```python
from build123d import *

# Parameters (mm, degrees)
F0_R     = 44.45
F0_R_2   = 6.35
F1_DEPTH = 3.175


with BuildPart() as f1:
    # F0 (on Top) → F1 (new body)
    with BuildSketch(Plane.XY):
        Circle(F0_R)
        with BuildLine():
            add(Edge.make_bspline(
                [(-20.4392500678, -2.7074250448), (-18.5086635833, -4.8096192168), (-18.5086635833, -8.1559691232)],
                knots=[0, 0, 0, 1, 1, 1], degree=2))
            add(Edge.make_bspline(
                [(-18.5086635833, -8.1559691232), (-18.5086635833, -12.4676122719), (-21.6369287203, -14.8844205377)],
                knots=[0, 0, 0, 1, 1, 1], degree=2))
            add(Edge.make_bspline(
                [(-21.6369287203, -14.8844205377), (-24.7651938572, -17.3012288034), (-30.1279340918, -17.3012288034)],
                knots=[0, 0, 0, 1, 1, 1], degree=2))
            add(Edge.make_bspline(
                [(-30.1279340918, -17.3012288034), (-35.9339941859, -17.3012288034), (-39.065834483, -15.7996615377)],
                knots=[0, 0, 0, 1, 1, 1], degree=2))
            Line((-39.065834483, -15.7996615377), (-39.065834483, -12.1386975375))
            add(Edge.make_bspline(
                [(-39.065834483, -12.1386975375), (-37.0494441547, -12.9824353344), (-34.6826881312, -13.475807436)],
                knots=[0, 0, 0, 1, 1, 1], degree=2))
            add(Edge.make_bspline(
                [(-34.6826881312, -13.475807436), (-32.3159321076, -13.9691795376), (-29.9920780059, -13.9691795376)],
                knots=[0, 0, 0, 1, 1, 1], degree=2))
            add(Edge.make_bspline(
                [(-29.9920780059, -13.9691795376), (-26.1952579197, -13.9691795376), (-24.2718217556, -12.5283899946)],
                knots=[0, 0, 0, 1, 1, 1], degree=2))
            add(Edge.make_bspline(
                [(-24.2718217556, -12.5283899946), (-22.3483855914, -11.0876004515), (-22.3483855914, -8.5134851389)],
                knots=[0, 0, 0, 1, 1, 1], degree=2))
            add(Edge.make_bspline(
                [(-22.3483855914, -8.5134851389), (-22.3483855914, -6.8188592247), (-23.0312411813, -5.7355856973)],
                knots=[0, 0, 0, 1, 1, 1], degree=2))
            add(Edge.make_bspline(
                [(-23.0312411813, -5.7355856973), (-23.7140967712, -4.6523121699), (-25.3121933611, -3.7334960097)],
                knots=[0, 0, 0, 1, 1, 1], degree=2))
            add(Edge.make_bspline(
                [(-25.3121933611, -3.7334960097), (-26.910289951, -2.8146798495), (-30.1708360137, -1.6563279588)],
                knots=[0, 0, 0, 1, 1, 1], degree=2))
            add(Edge.make_bspline(
                [(-30.1708360137, -1.6563279588), (-34.725590053, -0.0260549274), (-36.6812026586, 2.2084201704)],
                knots=[0, 0, 0, 1, 1, 1], degree=2))
            add(Edge.make_bspline(
                [(-36.6812026586, 2.2084201704), (-38.6368152642, 4.4428952681), (-38.6368152642, 8.0395063855)],
                knots=[0, 0, 0, 1, 1, 1], degree=2))
            add(Edge.make_bspline(
                [(-38.6368152642, 8.0395063855), (-38.6368152642, 11.8148755108), (-35.8017132601, 14.0493506086)],
                knots=[0, 0, 0, 1, 1, 1], degree=2))
            add(Edge.make_bspline(
                [(-35.8017132601, 14.0493506086), (-32.9666112561, 16.2838257063), (-28.2903017714, 16.2838257063)],
                knots=[0, 0, 0, 1, 1, 1], degree=2))
            add(Edge.make_bspline(
                [(-28.2903017714, 16.2838257063), (-23.4209336383, 16.2838257063), (-19.3309504193, 14.4962456281)],
                knots=[0, 0, 0, 1, 1, 1], degree=2))
            Line((-19.3309504193, 14.4962456281), (-20.5179035913, 11.1927976435))
            add(Edge.make_bspline(
                [(-20.5179035913, 11.1927976435), (-24.5649848884, 12.8874235577), (-28.3832559355, 12.8874235577)],
                knots=[0, 0, 0, 1, 1, 1], degree=2))
            add(Edge.make_bspline(
                [(-28.3832559355, 12.8874235577), (-31.4006911075, 12.8874235577), (-33.0988921819, 11.5932155811)],
                knots=[0, 0, 0, 1, 1, 1], degree=2))
            add(Edge.make_bspline(
                [(-33.0988921819, 11.5932155811), (-34.7970932562, 10.2990076044), (-34.7970932562, 7.9966044637)],
                knots=[0, 0, 0, 1, 1, 1], degree=2))
            add(Edge.make_bspline(
                [(-34.7970932562, 7.9966044637), (-34.7970932562, 6.3019785495), (-34.1714402288, 5.2151298619)],
                knots=[0, 0, 0, 1, 1, 1], degree=2))
            add(Edge.make_bspline(
                [(-34.1714402288, 5.2151298619), (-33.5457872014, 4.1282811744), (-32.0585205763, 3.2237656548)],
                knots=[0, 0, 0, 1, 1, 1], degree=2))
            add(Edge.make_bspline(
                [(-32.0585205763, 3.2237656548), (-30.5712539512, 2.3192501352), (-27.5109168573, 1.2252511273)],
                knots=[0, 0, 0, 1, 1, 1], degree=2))
            add(Edge.make_bspline(
                [(-27.5109168573, 1.2252511273), (-22.3698365523, -0.6052308728), (-20.4392500678, -2.7074250448)],
                knots=[0, 0, 0, 1, 1, 1], degree=2))
        make_face(mode=Mode.SUBTRACT)
        Polygon((-1.7697637308, 12.4441036983), (-1.7697637308, -16.8507586237), (-5.566583817, -16.8507586237), (-5.566583817, 12.4441036983), (-15.9130973098, 12.4441036983), (-15.9130973098, 15.819054886), (8.576749762, 15.819054886), (8.576749762, 12.4441036983), align=None, mode=Mode.SUBTRACT)
        with BuildLine():
            Line((34.3679551307, 15.819054886), (38.1647752168, 15.819054886))
            Line((38.1647752168, 15.819054886), (38.1647752168, -5.317291959))
            add(Edge.make_bspline(
                [(38.1647752168, -5.317291959), (38.1647752168, -10.9088424437), (34.7898240291, -14.1050356236)],
                knots=[0, 0, 0, 1, 1, 1], degree=2))
            add(Edge.make_bspline(
                [(34.7898240291, -14.1050356236), (31.4148728414, -17.3012288034), (25.5158585833, -17.3012288034)],
                knots=[0, 0, 0, 1, 1, 1], degree=2))
            add(Edge.make_bspline(
                [(25.5158585833, -17.3012288034), (19.6168443251, -17.3012288034), (16.3884747038, -14.0800095025)],
                knots=[0, 0, 0, 1, 1, 1], degree=2))
            add(Edge.make_bspline(
                [(16.3884747038, -14.0800095025), (13.1601050826, -10.8587902015), (13.1601050826, -5.2314881152)],
                knots=[0, 0, 0, 1, 1, 1], degree=2))
            Line((13.1601050826, -5.2314881152), (13.1601050826, 15.819054886))
            Line((13.1601050826, 15.819054886), (16.964075489, 15.819054886))
            Line((16.964075489, 15.819054886), (16.964075489, -5.4960499668))
            add(Edge.make_bspline(
                [(16.964075489, -5.4960499668), (16.964075489, -9.5860331858), (19.1985505868, -11.7776063617)],
                knots=[0, 0, 0, 1, 1, 1], degree=2))
            add(Edge.make_bspline(
                [(19.1985505868, -11.7776063617), (21.4330256846, -13.9691795376), (25.7661197942, -13.9691795376)],
                knots=[0, 0, 0, 1, 1, 1], degree=2))
            add(Edge.make_bspline(
                [(25.7661197942, -13.9691795376), (29.8990049351, -13.9691795376), (32.1334800329, -11.7668808812)],
                knots=[0, 0, 0, 1, 1, 1], degree=2))
            add(Edge.make_bspline(
                [(32.1334800329, -11.7668808812), (34.3679551307, -9.5645822249), (34.3679551307, -5.4531480449)],
                knots=[0, 0, 0, 1, 1, 1], degree=2))
            Line((34.3679551307, -5.4531480449), (34.3679551307, 15.819054886))
        make_face(mode=Mode.SUBTRACT)
        with Locations((0, 34.6494875848)):
            Circle(F0_R_2, mode=Mode.SUBTRACT)
    extrude(amount=F1_DEPTH)


solid = f1.part
```
Can you work these out from the model? Positions are in its coordinate system, mm. Give positions to 0.01 mm unless a question says otherwise; leave off trailing zeros. Loops run counter-clockwise (first coordinate to the right, second up) from the corner with the lowest first, then second, coordinate; pieces in that order, holes last. Notation, with made-up numbers: M 8.25,43.25 L 61.25,43.25 A26 ccw 61.25,68.25 Z; hole C 50,-3.75 d1. An arc over 180 degrees is marked long. One line per item, written item: value.
(1) Suppose I cut it at C-C on x = -11. List the corners of the cut face in (y, z) for me (3 decimals), plus the area to 3 significant figures.
Returned:
outline: M -43.067,0 L 12.444,0 L 12.444,3.175 L -43.067,3.175 Z; M 15.819,0 L 43.067,0 L 43.067,3.175 L 15.819,3.175 Z
area: 263 mm^2
(2) Suppose I cut it at B-B on y = 31.5. List the corners of the cut face in (x, z) for me (3 decimals), plus the area to 3 significant figures.
Returned:
outline: M -31.362,0 L -5.514,0 L -5.514,3.175 L -31.362,3.175 Z; M 5.514,0 L 31.362,0 L 31.362,3.175 L 5.514,3.175 Z
area: 164 mm^2
(3) Suppose I cut it at D-D on z = 0.6. Count the separate pieces of the cut face and the enclosed holes in it, plus the area to 3 significant figures.
Returned:
separate pieces: 1
enclosed holes: 4
area: 5,360 mm^2
(4) Will these pins go through, and if not, where does the flat tip stop? pin 1 (1.6 mm diameter, centred on y = 7, z = 1.5, fed in from -X); pin 2 (1 mm diameter, centred on y = 5.5, z = 1, fed in from +X); pin 3 (1.5 mm diameter, centred on y = 23.5, z = 2.5, fed in from -X).
Returned:
pin 1: x = -44.02
pin 2: x = 44.17
pin 3: x = -38.19
(5) I need wall thicknesses on line 1 (Y direction, x = 0, z = 2); line 2 (Y direction, x = -21, z = 0.7); line 3 (X direction, y = -10, z = 2.8). Which ranges of each line are inside material? Lowest first, please.
Returned:
line 1: -44.45 to 12.44, 15.82 to 28.3, 41 to 44.45
line 2: -39.18 to -14.34, -2.16 to 11.39, 15.14 to 39.18
line 3: -43.31 to -22.53, -18.67 to -5.57, -1.77 to 13.88, 17.9 to 33.42, 37.43 to 43.31
(6) Suppose I cut it at A-A on x = 0. List the corners of the cut face in (y, z) for me (3 decimals), plus the area to 3 significant figures.
Returned:
outline: M -44.45,0 L 12.444,0 L 12.444,3.175 L -44.45,3.175 Z; M 15.819,0 L 28.299,0 L 28.299,3.175 L 15.819,3.175 Z; M 40.999,0 L 44.45,0 L 44.45,3.175 L 40.999,3.175 Z
area: 231 mm^2
(7) We'd pull the mould along X, two halves only. Please class faces 1 (the face through (42.397, 13.352, 1.565)), 2 (the face through (-11, 12.444, 2)), 3 (the face through (-1, 1, 3.175)), 4 (the face through (13.16, 5, 2)): released by +X, released by -X, zero draft, split by the parting line, or undercut.
Returned:
face 1: split by the parting line
face 2: undercut
face 3: zero draft
face 4: undercut
